```python
from build123d import *

# Parameters (mm, degrees)
EXTRUDE_1_DEPTH     = 48
CUT_EXTRUDE_1_DEPTH = 66
CUT_EXTRUDE_2_DEPTH = 5
CUT_EXTRUDE_START   = -5
CUT_EXTRUDE_3_DEPTH = 5
CUT_EXTRUDE_5_DEPTH = 30
CUT_EXTRUDE_6_DEPTH = 30


with BuildPart() as part:
    # 草图1 → 凸台-拉伸1 (new body)
    with BuildSketch(Plane(origin=(0, 0, 0), x_dir=(1, 0, 0), z_dir=(0, 1, 0))):
        Polygon((10, 4.142135624), (4.142135624, 10), (-4.142135624, 10), (-10, 4.142135624), (-10, -4.142135624), (-4.142135624, -10), (4.142135624, -10), (10, -4.142135624), align=None)
    extrude(amount=EXTRUDE_1_DEPTH)

    # 草图2 → 切除-拉伸1 (cut)
    with BuildSketch(Plane.XY.offset(10)):
        with BuildLine():
            Line((-10, 10), (-10, -2.389295552))
            Line((-10, -2.389295552), (10, -2.389295552))
            Line((10, -2.389295552), (10, 10))
            ThreePointArc((10, 10), (0, 0), (-10, 10))
        make_face()
    extrude(amount=-CUT_EXTRUDE_1_DEPTH, mode=Mode.SUBTRACT)

    # 草图4 → 切除-拉伸2 (cut)
    with BuildSketch(Plane.XY.offset(10)):
        with BuildLine():
            Line((-10, 10), (-10, 20))
            Line((-10, 20), (10, 20))
            Line((10, 20), (10, 10))
            ThreePointArc((10, 10), (0, 0), (-10, 10))
        make_face()
    extrude(amount=-CUT_EXTRUDE_2_DEPTH, mode=Mode.SUBTRACT)

    # 草图5 → 切除-拉伸3 (cut)
    with BuildSketch(Plane(origin=(0, 0, -10), x_dir=(-1, 0, 0), z_dir=(0, 0, -1)).offset(CUT_EXTRUDE_START)):
        with BuildLine():
            Line((-10, 10), (-10, 20))
            Line((-10, 20), (10, 20))
            Line((10, 20), (10, 10))
            ThreePointArc((10, 10), (0, 0), (-10, 10))
        make_face()
    extrude(amount=CUT_EXTRUDE_3_DEPTH, mode=Mode.SUBTRACT)

    # 草图7 → 切除-拉伸5 (cut)
    with BuildSketch(Plane.XY.offset(10)):
        with BuildLine():
            Line((-10, 30), (-10, 50.94058397))
            Line((-10, 50.94058397), (10, 50.94058397))
            Line((10, 50.94058397), (10, 30))
            ThreePointArc((10, 30), (0, 40), (-10, 30))
        make_face()
    extrude(amount=-CUT_EXTRUDE_5_DEPTH, mode=Mode.SUBTRACT)

    # 草图8 → 切除-拉伸6 (cut)
    with BuildSketch(Plane(origin=(10, 0, 0), x_dir=(0, 0, -1), z_dir=(1, 0, 0))):
        with BuildLine():
            Line((-10, 30), (-10, 44.07560735))
            Line((-10, 44.07560735), (10, 44.07560735))
            Line((10, 44.07560735), (10, 30))
            ThreePointArc((10, 30), (0, 40), (-10, 30))
        make_face()
    extrude(amount=-CUT_EXTRUDE_6_DEPTH, mode=Mode.SUBTRACT)


solid = part.part
```
Geometry check sheet. Reference: the model listing, model coordinates, mm. A direction names the side the tool comes from. Give positions to 0.01 mm unless a question says otherwise; leave off trailing zeros. Write each loop counter-clockwise with the first axis right and the second up, starting at its lowest first coordinate (ties: lowest second). Pieces come first, ordered by that corner, then holes.
1) Access from +Z, -Z, +X, -X, +Y, -Y to the whole of each face (thin tool, end or side, straight path). Record for faces 1 (the flat face through (0, 20, 7)), 2 (the flat face through (0, 25, -10)), 3 (the flat face through (0, 20, -7)).
2) Section check D-D, the plane x = 6. Record the boundary of the cut face in (y, z).
3) Section check A-A, the plane y = 13.5. Record the boundary of the cut face in (x, z).
4) Gauge pin test, flat ends, axial feed: pin 1 (6 mm diameter, centred on x = -7.5, y = 4.5, fed in from +Z); pin 2 (8 mm diameter, centred on x = -3, y = 34.5, fed in from -Z); pin 3 (1 mm diameter, centred on y = 30.5, z = 6.5, fed in from -X). Record the tip position at first contact, or that the pin passes through.
5) Section check B-B, the plane x = 8.25. Record the boundary of the cut face in (y, z).
6) Section check C-C, the plane z = 6.5. Record the boundary of the cut face in (x, y), and give its area (3 significant figures).
7) Material ranges on L1, parallel to Z at x = -4.75, y = 9.5; L2, parallel to Z at x = 7.5, y = 29; L3, parallel to Y at x = 1.5, z = 8.5, recorded low to high.
Computed:
1. face 1: +Z, +X, -X, -Y
1. face 2: -Z, +X, -X, +Y, -Y
1. face 3: -Z, +X, -X, -Y
2. outline: (2, -5) - (20, -5) - (20, -8.14) - (35.81, -8.14) arc R10 ccw to (38, -6) - (38, 6) arc R10 ccw to (35.81, 8.14) - (20, 8.14) - (20, 5) - (2, 5) - close
3. outline: (-10, -4.14) - (-9.14, -5) - (9.14, -5) - (10, -4.14) - (10, 4.14) - (9.14, 5) - (-9.14, 5) - (-10, 4.14) - close
4. pin 1: stops at z = 5
4. pin 2: stops at z = -9.99
4. pin 3: stops at x = -8.14
5. outline: (4.35, -5) - (20, -5) - (20, -5.89) - (35.65, -5.89) - (35.65, 5.89) - (20, 5.89) - (20, 5) - (4.35, 5) - close
6. outline: (-7.64, 20) - (7.64, 20) - (7.64, 36.45) arc R10 ccw to (6.5, 37.6) - (-6.5, 37.6) arc R10 ccw to (-7.64, 36.45) - close
6. area: 268 mm2
7. L1: z = -5 to 5
7. L2: z = -6.64 to 6.64
7. L3: y = 20 to 35.27
